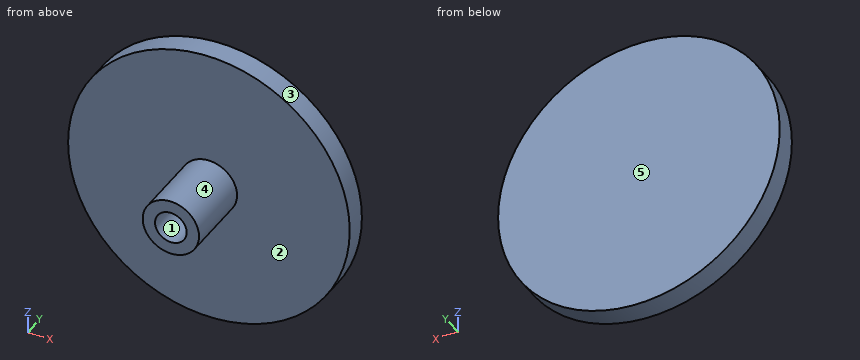
```python
from build123d import *

# Parameters (mm, degrees)
F0_R     = 15.875
F1_DEPTH = 2.54
F2_R     = 3.175
F2_R_2   = 1.785938
F3_DEPTH = 7.9375


with BuildPart() as f1:
    # F0 (on Front) → F1 (new body)
    with BuildSketch(Plane.XZ):
        Circle(F0_R)
    extrude(amount=F1_DEPTH)

    # F2 (on face) → F3 (join)
    with BuildSketch(Plane.XZ.offset(2.54)):
        Circle(F2_R)
        Circle(F2_R_2, mode=Mode.SUBTRACT)
    extrude(amount=F3_DEPTH)


solid = f1.part
```
Geometry: final body of the model. Coordinates: model frame, mm. Face numbers are marked on the shaded views. A direction names the side the tool comes from. Give positions to 0.01 mm unless a question says otherwise; leave off trailing zeros. Loops run counter-clockwise (first coordinate to the right, second up) from the corner with the lowest first, then second, coordinate; pieces in that order, holes last. Notation, with made-up numbers: (-10.75, 63.25) -> (28.25, 63.25) arc R16 cw to (28.25, 72.25) -> close; hole circle Ø3 at (-1.75, -3). An arc over 180 degrees is marked (long way). Use one line per item in the form item = value.
Item 1: Section query A-A on z = 0. Output: boundary loops of the cut face in (x, y) (1 decimal), and give its area (3 significant figures).
A:
outline = (-15.9, -2.5) -> (-3.2, -2.5) -> (-3.2, -10.5) -> (-1.8, -10.5) -> (-1.8, -2.5) -> (1.8, -2.5) -> (1.8, -10.5) -> (3.2, -10.5) -> (3.2, -2.5) -> (15.9, -2.5) -> (15.9, 0) -> (-15.9, 0) -> close
area = 103 mm^2
Item 2: Line query: probe 1 along Z at (x, y) = (0, -8.75) (3 decimals); probe 2 along Y at (x, z) = (-1.5, 4); probe 3 along Z at (x, y) = (-1, -5.75). Output: solid intervals per line, ascending.
A:
probe_1 = -3.175 to -1.786, 1.786 to 3.175
probe_2 = -2.54 to 0
probe_3 = -3.01 to -1.48, 1.48 to 3.01
Item 3: Access query for the marked faces 4 and 5. Directions: +Z, -Z, +X, -X, +Y, -Y. A direction counts if a zero-diameter tool reaches every point of the face in a straight line with its end or side. Return the directions, or none.
A:
face_4 = -Y
face_5 = +Z, -Z, +X, -X, +Y
Item 4: Section query B-B on x = 0. Output: boundary loops of the cut face in (y, z) (1 decimal), and give its area (3 significant figures).
A:
outline = (-10.5, -3.2) -> (-2.5, -3.2) -> (-2.5, -15.9) -> (0, -15.9) -> (0, 15.9) -> (-2.5, 15.9) -> (-2.5, 3.2) -> (-10.5, 3.2) -> (-10.5, 1.8) -> (-2.5, 1.8) -> (-2.5, -1.8) -> (-10.5, -1.8) -> close
area = 103 mm^2
Item 5: Section query D-D on x = -5. Output: boundary loops of the cut face in (y, z).
A:
outline = (-2.54, -15.07) -> (0, -15.07) -> (0, 15.07) -> (-2.54, 15.07) -> close
Item 6: Pin query (flat end, axial travel): P1, Ø3, axis at y = -1.5, z = -8, coming from the -X side; P2, Ø6, axis at x = 0.5, y = -2, coming from the +Z side (3 decimals); P3, Ø1.8, axis at x = 0, z = -0.5, coming from the -Y side; P4, Ø5, axis at y = -8, z = 2, coming from the -X side (3 decimals). Return the tip coordinate at first contact, or that it passes through.
A:
P1 = -14.48
P2 = 15.875
P3 = -2.54
P4 = -3.175
Item 7: Section query C-C on y = -7. Output: boundary loops of the cut face in (x, z) (3 decimals), and give its area (3 significant figures).
A:
outline = circle Ø6.35 at (0, 0); hole circle Ø3.572 at (0, 0)
area = 21.6 mm^2
Item 8: Draft query along X for the marked faces 1, 2 and 3. Return one class per face: pulls with the +X half, pulls with the -X half, needs draft (parallel to the pull), parting line crosses it, or undercut.
A:
face_1 = undercut
face_2 = needs draft
face_3 = parting line crosses it
